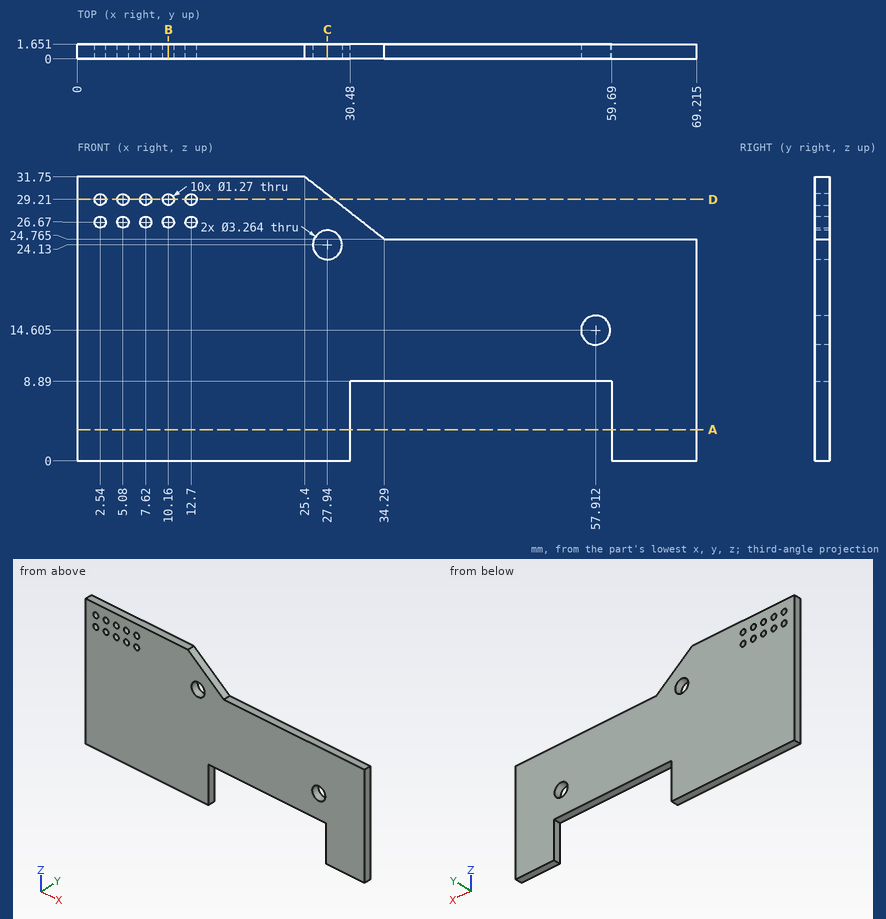
Here's the drawing with two shaded views (mm, measured from the low corner). I have some questions. Coordinates: 2 decimals unless noted, no trailing zeros. Write each loop counter-clockwise with the first axis right and the second up, starting at its lowest first coordinate (ties: lowest second). Pieces come first, ordered by that corner, then holes. Notation, with made-up numbers: (88.25, 7.5) -> (104.25, 7.5) arc R26 ccw to (104.25, 23.5) -> close; hole circle Ø7 at (12, 53.5). An arc over 180 degrees is marked (long way). Write item = value, one per line. Start each with the question number.
(1) I need wall thicknesses on line 1 (X direction, y = 0.9, z = 7.5) (3 decimals); line 2 (X direction, y = 1, z = 26.67) (1 decimal); line 3 (X direction, y = 0.75, z = 26.5). Which ranges of each line are inside material? Lowest first, please. Write a range as [from, to].
(2) I want a section at B-B (x = 10.16). Please give me the cut outline in (y, z) (3 decimals), plus the area to 3 significant figures.
(3) I want a section at D-D (z = 29.21). Please give me the cut outline in (x, y) (3 decimals), plus the area to 3 significant figures.
(4) I want a section at A-A (z = 3.5). Please give me the cut outline in (x, y) (3 decimals).
(5) I want a section at C-C (x = 27.94). Please give me the cut outline in (y, z), plus the area to 3 significant figures.
Result set:
q1.line_1 = [0, 30.48], [59.69, 69.215]
q1.line_2 = [0, 1.9], [3.2, 4.4], [5.7, 7], [8.3, 9.5], [10.8, 12.1], [13.3, 31.9]
q1.line_3 = [0, 1.93], [3.15, 4.47], [5.69, 7.01], [8.23, 9.55], [10.77, 12.09], [13.31, 32.08]
q2.outline = (0, 0) -> (1.651, 0) -> (1.651, 26.035) -> (0, 26.035) -> close; (0, 27.305) -> (1.651, 27.305) -> (1.651, 28.575) -> (0, 28.575) -> close; (0, 29.845) -> (1.651, 29.845) -> (1.651, 31.75) -> (0, 31.75) -> close
q2.area = 48.2 mm2
q3.outline = (0, 0) -> (1.905, 0) -> (1.905, 1.651) -> (0, 1.651) -> close; (3.175, 0) -> (4.445, 0) -> (4.445, 1.651) -> (3.175, 1.651) -> close; (5.715, 0) -> (6.985, 0) -> (6.985, 1.651) -> (5.715, 1.651) -> close; (8.255, 0) -> (9.525, 0) -> (9.525, 1.651) -> (8.255, 1.651) -> close; (10.795, 0) -> (12.065, 0) -> (12.065, 1.651) -> (10.795, 1.651) -> close; (13.335, 0) -> (28.633, 0) -> (28.633, 1.651) -> (13.335, 1.651) -> close
q3.area = 36.8 mm2
q4.outline = (0, 0) -> (30.48, 0) -> (30.48, 1.651) -> (0, 1.651) -> close; (59.69, 0) -> (69.215, 0) -> (69.215, 1.651) -> (59.69, 1.651) -> close
q5.outline = (0, 0) -> (1.65, 0) -> (1.65, 22.5) -> (0, 22.5) -> close; (0, 25.76) -> (1.65, 25.76) -> (1.65, 29.75) -> (0, 29.75) -> close
q5.area = 43.7 mm2
